```python
from build123d import *

# Parameters (mm, degrees)
SKETCH_R  = 1.822871
PAD_DEPTH = 1.6


with BuildPart() as part:
    # Sketch → Pad (new body)
    with BuildSketch(Plane.XY):
        Polygon((14, 16), (16, 14), (16, -14), (14, -16), (-14, -16), (-16, -14), (-16, 13.796185), (-14, 16), align=None)
        with Locations((-11.9, 12.032497)):
            Circle(SKETCH_R, mode=Mode.SUBTRACT)
        with Locations((12, 12.032497)):
            Circle(SKETCH_R, mode=Mode.SUBTRACT)
        with Locations((-11.852346, -11.872872)):
            Circle(SKETCH_R, mode=Mode.SUBTRACT)
        with Locations((12, -11.9)):
            Circle(SKETCH_R, mode=Mode.SUBTRACT)
        with BuildLine():
            ThreePointArc((3.984503, 4.492219), (0.062772, 6.004362), (-3.889715, 4.57454))
            Line((-3.889715, 4.57454), (-8.654236, 9.264053))
            Line((-8.654236, 9.264053), (-9.260711, 8.720268))
            Line((-9.260711, 8.720268), (-4.466236, 4.013607))
            ThreePointArc((-4.466236, 4.013607), (-6.00462, 0.029046), (-4.504856, -3.970211))
            Line((-9.309208, -8.743832), (-4.504856, -3.970211))
            Line((-8.762374, -9.368784), (-9.309208, -8.743832))
            Line((-3.901652, -4.564363), (-8.762374, -9.368784))
            ThreePointArc((-3.901652, -4.564363), (0.06724, -6.004314), (4.00289, -4.475843))
            Line((8.697231, -9.271135), (4.00289, -4.475843))
            Line((9.302653, -8.638371), (8.697231, -9.271135))
            Line((4.46051, -4.019969), (9.302653, -8.638371))
            ThreePointArc((4.46051, -4.019969), (6.004416, -0.057401), (4.536548, 3.933959))
            Line((9.274082, 8.77581), (4.536548, 3.933959))
            Line((8.727249, 9.244524), (9.274082, 8.77581))
            Line((3.984503, 4.492219), (8.727249, 9.244524))
        make_face(mode=Mode.SUBTRACT)
    extrude(amount=-PAD_DEPTH)


solid = part.part
```
CAD build for the part. Positions are in the model's coordinates, mm. A direction names the side the tool comes from. Give positions to 0.01 mm unless a question says otherwise; leave off trailing zeros. Loops run counter-clockwise (first coordinate to the right, second up) from the corner with the lowest first, then second, coordinate; pieces in that order, holes last. Notation, with made-up numbers: M -17.5,-19 L 39.5,-19 A19 ccw 39.5,-1 Z; hole C 89,15.5 d5. An arc over 180 degrees is marked long. Use one line per item in the form item = value.
Item 1: Slice it at C-C (z = -0.6). List the corners of the cut face in (x, y).
Determined:
outline = M -16,-14 L -14,-16 L 14,-16 L 16,-14 L 16,14 L 14,16 L -14,16 L -16,13.8 Z; hole C -11.9,12.03 d3.65; hole C -11.85,-11.87 d3.65; hole M -9.31,-8.74 L -8.76,-9.37 L -3.9,-4.56 A6 ccw 4,-4.48 L 8.7,-9.27 L 9.3,-8.64 L 4.46,-4.02 A6 ccw 4.54,3.93 L 9.27,8.78 L 8.73,9.24 L 3.98,4.49 A6 ccw -3.89,4.57 L -8.65,9.26 L -9.26,8.72 L -4.47,4.01 A6 ccw -4.5,-3.97 Z; hole C 12,-11.9 d3.65; hole C 12,12.03 d3.65
Item 2: Slice it at A-A (x = 12). List the corners of the cut face in (y, z), plus the area to 3 significant figures.
Determined:
outline = M -16,-1.6 L -13.72,-1.6 L -13.72,0 L -16,0 Z; M -10.08,-1.6 L 10.21,-1.6 L 10.21,0 L -10.08,0 Z; M 13.86,-1.6 L 16,-1.6 L 16,0 L 13.86,0 Z
area = 39.5 mm2
Item 3: Two-plate mould, pull along X, no slides. Class faces 3 (the face through (15, -15, -1)), 4 (the face through (6.94, 6.39, -0.79)), 5 (the face through (-7, 0, -1.6)): pulls with the +X half, pulls with the -X half, needs draft (parallel to the pull), parting line crosses it, or undercut.
Determined:
face_3 = pulls with the +X half
face_4 = undercut
face_5 = needs draft
Item 4: Which spindle directions (+Z, -Z, +X, -X, +Y, -Y) get a long thin tool onto all of the face, cutting with end or side? Do faces 1 (the face through (-6.94, -6.39, -0.79)), 2 (the face through (-15, 14.9, -0.8)). Say none if no direction does.
Determined:
face_1 = +Z, -Z
face_2 = +Z, -Z, -X, +Y
Item 5: Flat gauge pin, fed straight in: pin 1 (3.5 mm diameter, centred on x = 12, y = 12.03, fed in from -Z). Where does the tip first touch, or does it go through?
Determined:
pin_1 = through
Item 6: Slice it at B-B (y = 6.5). List the corners of the cut face in (x, z).
Determined:
outline = M -16,-1.6 L -7,-1.6 L -7,0 L -16,0 Z; M -5.85,-1.6 L 5.99,-1.6 L 5.99,0 L -5.85,0 Z; M 7.05,-1.6 L 16,-1.6 L 16,0 L 7.05,0 Z
Item 7: Drill centre lines: probe 1 along Y at (x, z) = (12, -1); probe 2 along X at (y, z) = (8.5, -1.4); probe 3 along X at (y, z) = (-8.5, -0.75). Where is each one in solid material? Low to high. Write a range as from..to.
Determined:
probe_1 = -16..-13.72, -10.08..10.21, 13.86..16
probe_2 = -16..-9.04, -7.88..7.98, 9..16
probe_3 = -16..-9.06, -7.88..7.94, 9.16..16
